```python
from build123d import *

# Parameters (mm, degrees)
SKETCH1_R           = 8
BOSS_EXTRUDE1_DEPTH = 7
SKETCH2_R           = 6.8
CUT_EXTRUDE1_DEPTH  = 4
CUT_EXTRUDE2_DEPTH  = 4
SKETCH5_W           = 3
SKETCH5_H           = 3
CUT_EXTRUDE4_DEPTH  = 13


with BuildPart() as part:
    # Sketch1 → Boss-Extrude1 (new body)
    with BuildSketch(Plane.XY):
        with Locations(Location((0, 0, 0), (0, 0, 180))):
            Circle(SKETCH1_R)
    extrude(amount=BOSS_EXTRUDE1_DEPTH)

    # Sketch2 → Cut-Extrude1 (cut)
    with BuildSketch(Plane.XY.offset(7)):
        Circle(SKETCH2_R)
    extrude(amount=-CUT_EXTRUDE1_DEPTH, mode=Mode.SUBTRACT)

    # Sketch3 → Cut-Extrude2 (cut)
    with BuildSketch(Plane.XY):
        Polygon((4.67653718, 0), (2.33826859, 4.05), (-2.33826859, 4.05), (-4.67653718, 0), (-2.33826859, -4.05), (2.33826859, -4.05), align=None)
    extrude(amount=CUT_EXTRUDE2_DEPTH, mode=Mode.SUBTRACT)

    # Sketch5 → Cut-Extrude4 (cut, through all)
    with BuildSketch(Plane.XY.offset(3)):
        with Locations((0, 5.25)):
            Rectangle(SKETCH5_W, SKETCH5_H)
        with Locations((0, -5.25)):
            Rectangle(SKETCH5_W, SKETCH5_H)
    extrude(amount=-CUT_EXTRUDE4_DEPTH, mode=Mode.SUBTRACT)


solid = part.part
```
The listing builds one solid part. Answer for the finished solid, in the listing's coordinates (mm). A direction names the side the tool comes from. Give positions to 0.01 mm unless a question says otherwise; leave off trailing zeros. Order: outer loops, then holes, each group sorted by start corner. A loop starts at its lowest first (then second) coordinate and runs counter-clockwise, first axis right, second up. Notation, with made-up numbers: (19.5, 20.25) -> (26.5, 20.25) arc R15 cw to (26.5, 41.25) -> close; hole circle Ø3 at (51, 53.25). An arc over 180 degrees is marked (long way). Write each question's results on one line, items separated by ' | '.
Q1. The part is cut by section B-B, the plane y = 4.5. Give the vertices of the cut face in (x, z).
Checked values:
outline: (-6.61, 0) -> (-1.5, 0) -> (-1.5, 3) -> (-5.1, 3) -> (-5.1, 7) -> (-6.61, 7) -> close; (1.5, 0) -> (6.61, 0) -> (6.61, 7) -> (5.1, 7) -> (5.1, 3) -> (1.5, 3) -> close
Q2. The part is cut by section D-D, the plane x = 5.75. Give the vertices of the cut face in (y, z).
Checked values:
outline: (-5.56, 0) -> (5.56, 0) -> (5.56, 7) -> (3.63, 7) -> (3.63, 3) -> (-3.63, 3) -> (-3.63, 7) -> (-5.56, 7) -> close
Q3. The part is cut by section C-C, the plane z = 2.5. Give the vertices of the cut face in (x, y), and give its area (3 significant figures).
Checked values:
outline: circle Ø16 at (0, 0); hole (-4.68, 0) -> (-2.34, -4.05) -> (-1.5, -4.05) -> (-1.5, -6.75) -> (1.5, -6.75) -> (1.5, -4.05) -> (2.34, -4.05) -> (4.68, 0) -> (2.34, 4.05) -> (1.5, 4.05) -> (1.5, 6.75) -> (-1.5, 6.75) -> (-1.5, 4.05) -> (-2.34, 4.05) -> close | area: 128 mm^2
Q4. The part is cut by section A-A, the plane x = 0. Give the vertices of the cut face in (y, z), and give its area (3 significant figures).
Checked values:
outline: (-8, 0) -> (-6.75, 0) -> (-6.75, 3) -> (-6.8, 3) -> (-6.8, 7) -> (-8, 7) -> close; (6.75, 0) -> (8, 0) -> (8, 7) -> (6.8, 7) -> (6.8, 3) -> (6.75, 3) -> close | area: 17.1 mm^2
Q5. Which of the six approach directions +Z, -Z, +X, -X, +Y, -Y give full straight-line access (tool end or side, diameter ignored) to faces 1 (the face through (5, 0, 3)), 2 (the face through (0, -6.75, 2)), 3 (the face through (-3.491, 2.053, 1.479))?
Checked values:
face 1: +Z | face 2: -Z | face 3: +Z, -Z
Q6. Determine the mould class of faces 4 (the face through (1.5, 5, 2)), 5 (the face through (4, 6, 7)), 6 (the face through (1.73, 7.81, 3.45)) for opening direction Y: pulls with the +Y half, pulls with the -Y half, needs draft (parallel to the pull), parting line crosses it, or undercut.
Checked values:
face 4: undercut | face 5: needs draft | face 6: parting line crosses it
Q7. Straight lines are drawn through the part: probe 1 along Y at (x, z) = (0, 4.95); probe 2 along Y at (x, z) = (1, 5); probe 3 along X at (y, z) = (4.5, 4). For each, find the intervals that lie inside material, in ascending order. Write a range as from..to.
Checked values:
probe 1: y = -8..-6.8, 6.8..8 | probe 2: y = -7.94..-6.73, 6.73..7.94 | probe 3: x = -6.61..-5.1, 5.1..6.61
Q8. Each of these flat-tipped pins is pushed along its axis until it touches: P1, Ø1, axis at x = -2, y = -2.5, coming from the +Z side; P2, Ø0.7, axis at x = -2, z = 2, coming from the +Y side; P3, Ø3, axis at x = -6, z = 4, coming from the -Y side; P4, Ø2.5, axis at x = 5, y = 0.5, coming from the +Z side. Where does it stop, or does it pass through?
Checked values:
P1: passes through | P2: stops at y = 7.83 | P3: stops at y = -6.61 | P4: stops at z = 3
